Read the model definition and answer for the solid it produces. Units are mm, in the model's axes. Coordinates: 2 decimals unless noted, no trailing zeros. Write each loop counter-clockwise with the first axis right and the second up, starting at its lowest first coordinate (ties: lowest second). Pieces come first, ordered by that corner, then holes. Notation, with made-up numbers: (-7.75, -37) - (35.25, -37) arc R24 cw to (35.25, -20) - close; hole circle Ø5 at (83.25, 0.25). An arc over 180 degrees is marked (long way). Use a Markdown table: item, result.
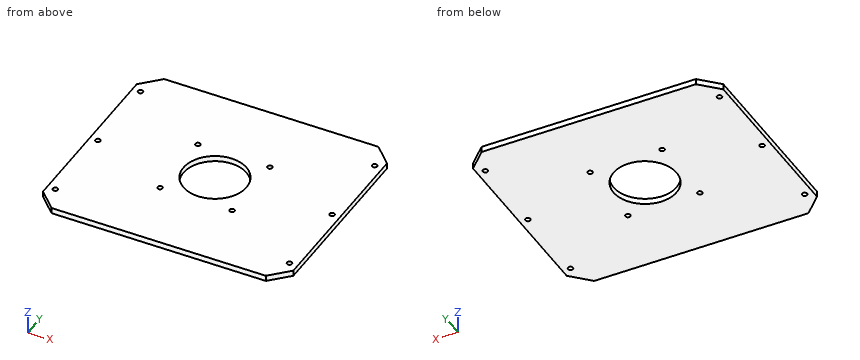
from build123d import *

# Parameters (mm, degrees)
SKETCH1_W           = 278
SKETCH1_H           = 238
BOSS_EXTRUDE1_DEPTH = 6.35
SKETCH2_R           = 35
SKETCH2_R_2         = 2.75
CUT_EXTRUDE1_DEPTH  = 7.35
CHAMFER1_SIZE       = 20
SKETCH4_R           = 2.75
CUT_EXTRUDE2_DEPTH  = 76.2


with BuildPart() as part:
    # Sketch1 → Boss-Extrude1 (new body)
    with BuildSketch(Plane.XY):
        Rectangle(SKETCH1_W, SKETCH1_H)
    extrude(amount=BOSS_EXTRUDE1_DEPTH)

    # Sketch2 → Cut-Extrude1 (cut, through all)
    with BuildSketch(Plane.XY.offset(6.35)):
        Circle(SKETCH2_R)
        with Locations((-40, 40)):
            Circle(SKETCH2_R_2)
        with Locations((40, 40)):
            Circle(SKETCH2_R_2)
        with Locations((40, -40)):
            Circle(SKETCH2_R_2)
        with Locations((-40, -40)):
            Circle(SKETCH2_R_2)
    extrude(amount=-CUT_EXTRUDE1_DEPTH, mode=Mode.SUBTRACT)

    # Chamfer1
    chamfer1_edges = [part.edges().sort_by_distance(p)[0] for p in [
        (-139, 119, 3.175),
        (139, 119, 3.175),
        (139, -119, 3.175),
        (-139, -119, 3.175),
    ]]
    chamfer(chamfer1_edges, length=CHAMFER1_SIZE)

    # Sketch4 → Cut-Extrude2 (cut)
    with BuildSketch(Plane.XY.offset(6.35)):
        with Locations((-130, 90)):
            Circle(SKETCH4_R)
        with Locations((130, 90)):
            Circle(SKETCH4_R)
        with Locations((-130, -90)):
            Circle(SKETCH4_R)
        with Locations((130, -90)):
            Circle(SKETCH4_R)
        with Locations((-130, 0)):
            Circle(SKETCH4_R)
        with Locations((130, 0)):
            Circle(SKETCH4_R)
    extrude(amount=-CUT_EXTRUDE2_DEPTH, mode=Mode.SUBTRACT)


solid = part.part
(1) Straight lines are drawn through the part: L1, parallel to X at y = -2, z = 2.25; L2, parallel to X at y = 88, z = 2; L3, parallel to Y at x = -130, z = 3.75. For each, find the intervals that lie inside material, in ascending order.
Report:
| item | result |
|---|---|
| L1 | x = -139 to -131.89, -128.11 to -34.94, 34.94 to 128.11, 131.89 to 139 |
| L2 | x = -139 to -131.89, -128.11 to 128.11, 131.89 to 139 |
| L3 | y = -108 to -92.75, -87.25 to -2.75, 2.75 to 87.25, 92.75 to 108 |
(2) This flat-tipped pin is pushed along its axis until it touches: P1, Ø5, axis at x = 130, y = 0, coming from the -Z side. Where does it stop, or does it pass through?
Report:
| item | result |
|---|---|
| P1 | passes through |
(3) A cutting plane is placed at B-B, the plane x = 0. Write down the section's boundary in (y, z), and give its area (3 significant figures).
Report:
| item | result |
|---|---|
| outline | (-119, 0) - (-35, 0) - (-35, 6.35) - (-119, 6.35) - close; (35, 0) - (119, 0) - (119, 6.35) - (35, 6.35) - close |
| area | 1,070 mm² |
(4) A cutting plane is placed at A-A, the plane z = 5. Count the separate pieces of the cut face and the enclosed holes in it, and give its area (3 significant figures).
Report:
| item | result |
|---|---|
| separate pieces | 1 |
| enclosed holes | 11 |
| area | 61,300 mm² |
